Study the drawing (mm; zero at the part's minimum x, y, z) and answer. Coordinates: 2 decimals unless noted, no trailing zeros. Loops run counter-clockwise (first coordinate to the right, second up) from the corner with the lowest first, then second, coordinate; pieces in that order, holes last. Notation, with made-up numbers: (15, 35.5) - (71, 35.5) arc R27 ccw to (71, 67.5) - close; hole circle Ø8 at (45.25, 64). An arc over 180 degrees is marked (long way). Use one line per item in the form item = value. Start each with the question number.
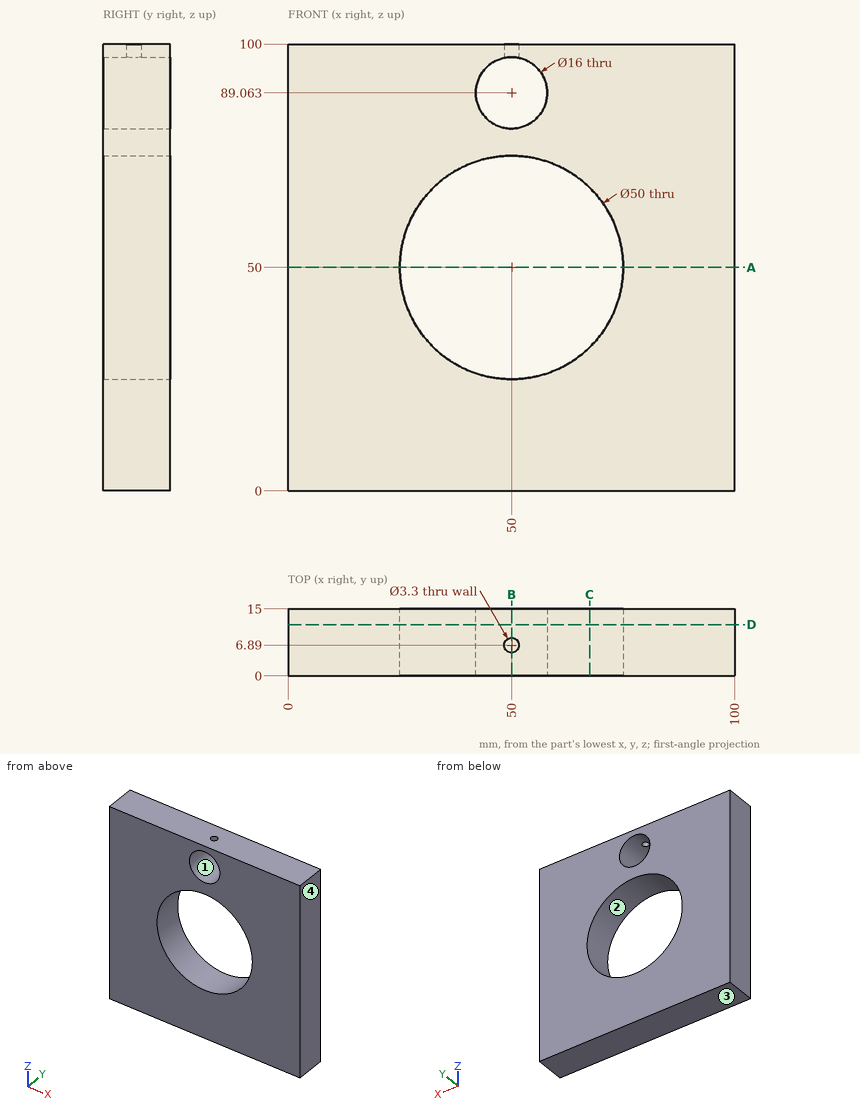
(1) A cutting plane is placed at C-C (x = 67.5). Determine the outline of the cut face in (y, z).
(2) Determine the mould class of the marked faces 1, 2, 3 and 4 for opening direction Z: +Z half, -Z half, draft (parallel to the pull), parting line (faces both ways), or undercut.
(3) A cutting plane is placed at D-D (y = 11.5). Determine the outline of the cut face in (x, z).
(4) A cutting plane is placed at A-A (z = 50). Determine the outline of the cut face in (x, y).
(5) A cutting plane is placed at B-B (x = 50). Determine the outline of the cut face in (y, z).
(6) Find the intervals of material crossed by probe 1 along Z at (x, y) = (50, 10); probe 2 along X at (y, z) = (5, 50); probe 3 along Y at (x, z) = (50, 98), in increasing order. Write a range as from..to.
Evaluation:
q1.outline = (0, 0) - (15, 0) - (15, 32.15) - (0, 32.15) - close; (0, 67.85) - (15, 67.85) - (15, 100) - (0, 100) - close
q2.face_1 = undercut
q2.face_2 = undercut
q2.face_3 = -Z half
q2.face_4 = draft
q3.outline = (0, 0) - (100, 0) - (100, 100) - (0, 100) - close; hole circle Ø50 at (50, 50); hole circle Ø16 at (50, 89.06)
q4.outline = (0, 0) - (25, 0) - (25, 15) - (0, 15) - close; (75, 0) - (100, 0) - (100, 15) - (75, 15) - close
q5.outline = (0, 0) - (15, 0) - (15, 25) - (0, 25) - close; (0, 75) - (15, 75) - (15, 81.06) - (0, 81.06) - close; (0, 97.06) - (5.24, 97.06) - (5.24, 100) - (0, 100) - close; (8.54, 97.06) - (15, 97.06) - (15, 100) - (8.54, 100) - close
q6.probe_1 = 0..25, 75..81.06, 97.06..100
q6.probe_2 = 0..25, 75..100
q6.probe_3 = 0..5.24, 8.54..15
